Build history of the part. All positions in model axes, mm. A direction names the side the tool comes from. Give positions to 0.01 mm unless a question says otherwise; leave off trailing zeros. Order: outer loops, then holes, each group sorted by start corner. A loop starts at its lowest first (then second) coordinate and runs counter-clockwise, first axis right, second up. Notation, with made-up numbers: (-33.75, 71.5) - (5.25, 71.5) arc R20 cw to (5.25, 94.5) - close; hole circle Ø9 at (24, 76). An arc over 180 degrees is marked (long way). Write each question's results on one line, items separated by ' | '. Start each with the question number.
1) Cut at B-B on y = -80. List the corners of the cut face in (x, z).
2) Two-plate mould, pull along Z, no slides. Class faces 1 (the face through (-2.17, 10.14, 49.76)), 2 (the face through (0, 20, 4)), 3 (the face through (-17.15, 10.14, 56.99)): +Z half, -Z half, draft (parallel to the pull), parting line (faces both ways), or undercut.
3) Drill centre lines: line 1 along X through (y, z) = (13, 40); line 2 along Z through (x, y) = (0, 4); line 3 along Y through (x, z) = (-12, -44). Where is each one in solid material? Low to high. Write a range as from..to.
4) Tool access for faces 4 (the face through (16.99, -97.15, -54.93)), 5 (the face through (0, -25, -45)): list every direction of +Z, -Z, +X, -X, +Y, -Y with a clear straight run to the whole face (end or side of a thin tool).
5) Cut at C-C on z = 40. List the corners of the cut face in (x, y).
6) Drop flat-ended pins along their axis: pin 1 Ø16.5 at (x, y) = (5, -19.5) entering from +Z; pin 2 Ø5 at (x, z) = (2.5, -43) entering from -Y. Give the stop position or say it passes through.
7) Cut at D-D on y = 12. List the corners of the cut face in (x, z), plus the area to 3 significant figures.
8) Cut at A-A on x = 0. List the corners of the cut face in (y, z), plus the area to 3 significant figures.
from build123d import *

# Parameters (mm, degrees)
SKETCH1_W           = 40
SKETCH1_H           = 120
BOSS_EXTRUDE1_DEPTH = 20
SKETCH3_W           = 40
SKETCH3_H           = 20
BOSS_EXTRUDE3_DEPTH = 100
SKETCH4_W           = 40
SKETCH4_H           = 75
CUT_EXTRUDE1_DEPTH  = 10
FILLET1_R           = 10
CUT_EXTRUDE2_REACH  = 122
SKETCH5_R           = 13.5
CUT_EXTRUDE3_REACH  = 122
SKETCH6_R           = 10
FILLET2_R           = 10


with BuildPart() as part:
    # Sketch1 → Boss-Extrude1 (new body)
    with BuildSketch(Plane(origin=(0, 0, 0), x_dir=(1, 0, 0), z_dir=(0, 1, 0))):
        Rectangle(SKETCH1_W, SKETCH1_H)
    extrude(amount=BOSS_EXTRUDE1_DEPTH)

    # Sketch3 → Boss-Extrude3 (add)
    with BuildSketch(Plane.XZ):
        with Locations((0, -50)):
            Rectangle(SKETCH3_W, SKETCH3_H)
    extrude(amount=BOSS_EXTRUDE3_DEPTH)

    # Sketch4 → Cut-Extrude1 (cut)
    with BuildSketch(Plane.XY.offset(-40)):
        with Locations((0, -62.5)):
            Rectangle(SKETCH4_W, SKETCH4_H)
    extrude(amount=-CUT_EXTRUDE1_DEPTH, mode=Mode.SUBTRACT)

    # Fillet1
    fillet1_edges = [part.edges().sort_by_distance(p)[0] for p in [
        (20, 10, 60),
        (-20, 10, 60),
        (20, -100, -55),
        (-20, -100, -55),
        (0, 20, -60),
    ]]
    fillet(fillet1_edges, radius=FILLET1_R)

    # Sketch5 → Cut-Extrude2 (cut, up to next)
    with BuildSketch(Plane(origin=(0, 0, -60), x_dir=(-1, 0, 0), z_dir=(0, 0, -1)), mode=Mode.PRIVATE) as cut_extrude2_sk1:
        with Locations((0, -80)):
            Circle(SKETCH5_R)
    cut_extrude2_tool1 = extrude(cut_extrude2_sk1.sketch, amount=-CUT_EXTRUDE2_REACH, mode=Mode.PRIVATE) & part.part
    add(cut_extrude2_tool1.solids().sort_by_distance((0, -80, -60))[0], mode=Mode.SUBTRACT)

    # Sketch6 → Cut-Extrude3 (cut, up to next)
    with BuildSketch(Plane(origin=(0, 20, 0), x_dir=(1, 0, 0), z_dir=(0, 1, 0)), mode=Mode.PRIVATE) as cut_extrude3_sk1:
        with Locations((0, -40)):
            Circle(SKETCH6_R)
    cut_extrude3_tool1 = extrude(cut_extrude3_sk1.sketch, amount=-CUT_EXTRUDE3_REACH, mode=Mode.PRIVATE) & part.part
    add(cut_extrude3_tool1.solids().sort_by_distance((0, 20, 40))[0], mode=Mode.SUBTRACT)

    # Fillet2
    fillet2_edges = [part.edges().sort_by_distance(p)[0] for p in [
        (0, 0, -40),
    ]]
    fillet(fillet2_edges, radius=FILLET2_R)


solid = part.part
Results:
1) outline: (-20, -60) - (-13.5, -60) - (-13.5, -50) - (-20, -50) - close; (13.5, -60) - (20, -60) - (20, -50) - (13.5, -50) - close
2) face 1: undercut | face 2: draft | face 3: +Z half
3) line 1: -20..-10, 10..20 | line 2: -60..30, 50..60 | line 3: -25..20
4) face 4: +Z, -Z, +X, -Y | face 5: +Z, +X, -X, -Y
5) outline: (-20, 0) - (-10, 0) - (-10, 20) - (-20, 20) - close; (10, 0) - (20, 0) - (20, 20) - (10, 20) - close
6) pin 1: z = -40 | pin 2: y = -25
7) outline: (-20, -59.8) - (20, -59.8) - (20, 50) arc R10 ccw to (10, 60) - (-10, 60) arc R10 ccw to (-20, 50) - close; hole circle Ø20 at (0, 40) | area: 4,430 mm^2
8) outline: (-100, -60) - (-93.5, -60) - (-93.5, -50) - (-100, -50) - close; (-66.5, -60) - (10, -60) arc R10 ccw to (20, -50) - (20, 30) - (0, 30) - (0, -30) arc R10 cw to (-10, -40) - (-25, -40) - (-25, -50) - (-66.5, -50) - close; (0, 50) - (20, 50) - (20, 60) - (0, 60) - close | area: 2,980 mm^2
